from build123d import *

# Parameters (mm, degrees)
F0_W     = 10.922
F0_H     = 28.702
F0_W_2   = 52.578
F0_H_2   = 10.922
F0_R     = 7.874
F1_DEPTH = 10.922
F2_DEPTH = 44.45
F3_SIZE2 = 52.628408
F3_SIZE  = 33.52799
F4_SIZE2 = 15.3979316793
F4_SIZE  = 26.67


# Not quite as in the source:
# - a fillet or chamfer is up to 0.001 mm smaller than in the source, because OpenCascade refuses the exact size


with BuildPart() as f1:
    # F0 (on Front) → F1 (new body)
    with BuildSketch(Plane.XZ):
        with Locations((-40.1902680954, 6.35)):
            Rectangle(F0_W, F0_H)
        with Locations((-8.4402680954, -24.638)):
            Rectangle(F0_W_2, F0_H_2)
        Polygon((-13.9012680954, 30.099), (-45.6512680954, 30.099), (-45.6512680954, 20.701), (-34.7292680954, 20.701), (-34.7292680954, -8.001), (-34.7292680954, -19.177), (17.8487319046, -19.177), (17.8487319046, -30.099), (81.3487319046, -30.099), (81.3487319046, 4.5768394209), align=None)
        with Locations((62.2987319046, -11.049)):
            Circle(F0_R, mode=Mode.SUBTRACT)
        Polygon((-34.7292680954, -8.001), (-45.6512680954, -8.001), (-45.6512680954, -30.099), (-34.7292680954, -30.099), (-34.7292680954, -19.177), align=None)
    extrude(amount=F1_DEPTH)

    # F0 (on Front) → F2 (join)
    with BuildSketch(Plane.XZ):
        with Locations((-40.1902680954, 6.35)):
            Rectangle(F0_W, F0_H)
        with Locations((-8.4402680954, -24.638)):
            Rectangle(F0_W_2, F0_H_2)
        Polygon((-34.7292680954, -8.001), (-45.6512680954, -8.001), (-45.6512680954, -30.099), (-34.7292680954, -30.099), (-34.7292680954, -19.177), align=None)
    extrude(amount=F2_DEPTH)

    # F3 (size 33.528 and 52.6284180296 in the source; OpenCascade refuses exactly that, so slightly less here)
    f3_edges = [f1.edges().sort_by_distance(p)[0] for p in [
        (17.848732, -44.45, -24.638),
    ]]
    f3_side = f1.faces().sort_by_distance((17.848732, -27.686, -24.638))[0]
    chamfer(f3_edges, length=F3_SIZE, length2=F3_SIZE2, reference=f3_side)

    # F4
    f4_edges = [f1.edges().sort_by_distance(p)[0] for p in [
        (-40.215472, -44.45, 20.701),
    ]]
    f4_side = f1.faces().sort_by_distance((-40.19028, -27.685963, 20.701))[0]
    chamfer(f4_edges, length=F4_SIZE, length2=F4_SIZE2, reference=f4_side)


solid = f1.part
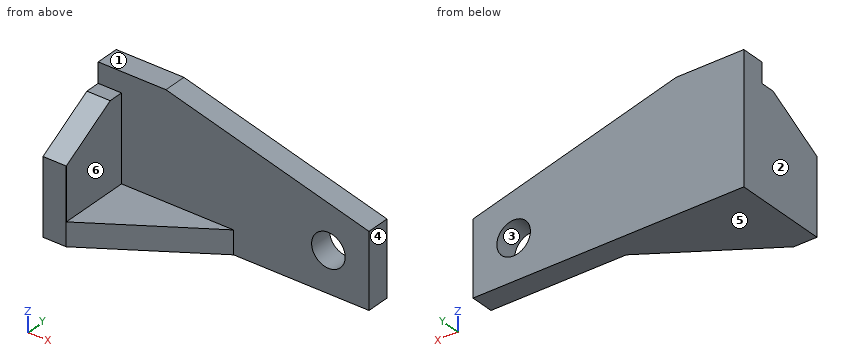
Design review of the part built by this model. Coordinates are the model's own, in mm. Face numbers are marked on the shaded views. A direction names the side the tool comes from. Coordinates: 2 decimals unless noted, no trailing zeros. Order: outer loops, then holes, each group sorted by start corner. A loop starts at its lowest first (then second) coordinate and runs counter-clockwise, first axis right, second up. Notation, with made-up numbers: M 81.25,28 L 95.25,28 A12 ccw 95.25,45 Z; hole C 38.5,-1.75 d3. An arc over 180 degrees is marked long. Use a Markdown table: item, result.
(1) For P1, Ø4, axis at y = -19.5, z = -5, coming from the +X side; P2, Ø8, axis at x = -3, z = -22.5, coming from the -Y side; P3, Ø10, axis at x = -8.5, y = -27, coming from the +Z side, all flat-tipped, find the tip position at first contact; note any pin that passes through.
Worked answers:
| item | result |
|---|---|
| P1 | stops at x = -34.73 |
| P2 | stops at y = -26.75 |
| P3 | stops at z = -19.18 |
(2) Add section C-C (x = 5). Give the boundary of the cut face in (y, z).
Worked answers:
| item | result |
|---|---|
| outline | M -19.11,-30.1 L 0,-30.1 L 0,25.03 L -10.92,25.03 L -10.92,-19.18 L -19.11,-19.18 Z |
(3) Wall thickness on probe 1 along Y at (x, z) = (-19, -14.5); probe 2 along X at (y, z) = (-25.5, 7); probe 3 along Z at (x, y) = (-20.5, -32): over which ranges is each line inside the solid? List them lowest first.
Worked answers:
| item | result |
|---|---|
| probe 1 | y = -10.92 to 0 |
| probe 2 | x = -45.65 to -34.73 |
| probe 3 | z = -30.1 to -19.18 |
(4) Draft analysis for pull direction X (two halves, no side actions). For the marked faces 1, 2, 3 and 4, state which applies: released by +X, released by -X, zero draft, split by the parting line, or undercut.
Worked answers:
| item | result |
|---|---|
| face 1 | zero draft |
| face 2 | released by -X |
| face 3 | undercut |
| face 4 | released by +X |
(5) Add section A-A (z = 0). Give the boundary of the cut face in (x, y).
Worked answers:
| item | result |
|---|---|
| outline | M -45.65,-44.45 L -34.78,-44.45 L -34.73,-44.42 L -34.73,-10.92 L 81.35,-10.92 L 81.35,0 L -45.65,0 Z |
(6) Add section B-B (y = -7.5). Give the boundary of the cut face in (x, z), then the cut area to 3 significant figures.
Worked answers:
| item | result |
|---|---|
| outline | M -45.65,-30.1 L 81.35,-30.1 L 81.35,4.58 L -13.9,30.1 L -45.65,30.1 Z; hole C 62.3,-11.05 d15.75 |
| area | 6,230 mm2 |
(7) Add section D-D (y = -38.5). Give the boundary of the cut face in (x, z), then the cut area to 3 significant figures.
Worked answers:
| item | result |
|---|---|
| outline | M -45.65,-30.1 L -25.44,-30.1 L -25.44,-19.18 L -34.73,-19.18 L -34.73,8.74 L -45.65,8.74 Z |
| area | 526 mm2 |
(8) For the marked faces 5 and 6, list the 3-axis set-ups (+Z, -Z, +X, -X, +Y, -Y) from which the entire face can be reached by the end or side of a thin tool; tool diameter is ignored.
Worked answers:
| item | result |
|---|---|
| face 5 | -Z, +X, -X, +Y, -Y |
| face 6 | +Z, +X, -Y |
